Autodesk Inventor part; units mm, degrees
ref_plane "ANBAU_XY" through (0, 0, 0) normal (0, 0, 1) x (1, 0, 0)
ref_plane "ANBAU_YZ" through (0, 0, 0) normal (1, 0, 0) x (0, 1, 0)
ref_plane "ANBAU_ZX" through (0, 0, 0) normal (0, 1, 0) x (0, 0, 1)
sketch "Sketch_1" plane through (0, 0, 0) normal (1, 0, 0) x (0, 1, 0)
  line L0 (0, -19) -> (0, 0)
  line L1 (23, 0) -> (23, -8.65)
  arc A0 (22.6, -9.05) -> (23, -8.65) centre (22.6, -8.65) ccw
  line L2 (22.6, -9.05) -> (16.6, -9.05)
  line L3 (16.6, -9.05) -> (16, -9.65)
  line L4 (16, -9.65) -> (16, -19)
  line L5 (16, -19) -> (37.4, -19)
  line L6 (37.4, -19) -> (39, -17.4)
  line L7 (39, -17.4) -> (39, 0)
  line L8 (39, 0) -> (23, 0)
revolve "Revolution1" add sketch "Sketch_1" angle 360 about axis through (0, 0, -19) along (0, 0, -1)
sketch "Sketch_2" plane through (0, 0, 0) normal (1, 0, 0) x (0, 1, 0)
  line L0 (31, -19) -> (31, 0)
  line L1 (31, 0) -> (37, 0)
  line L2 (37, 0) -> (36.053, -0.947)
  line L3 (36.053, -0.947) -> (36.053, -18.053)
  line L4 (36.053, -18.053) -> (37, -19)
  line L5 (37, -19) -> (31, -19)
  line L6 (31, -19) -> (31, 0)
revolve "Revolution2" cut sketch "Sketch_2" angle 360 about axis through (0, 31, -19) along (0, 0, -1)
thread "Thread1"
pattern_linear "Rectangular Pattern1" count 2 spacing 43.8406 along (-0.7071, -0.7071, 0) count 2 spacing 43.8406 along (0.7071, -0.7071, 0) of "Revolution2"
ref_plane "ANBAU_XY" through (0, 0, 0) normal (0, 0, 1) x (1, 0, 0)
ref_plane "ANBAU_YZ" through (0, 0, 0) normal (1, 0, 0) x (0, 1, 0)
ref_plane "ANBAU_ZX" through (0, 0, 0) normal (0, 1, 0) x (0, 0, 1)
ref_plane "EP_IP_XY" through (0, 0, -9.05) normal (0, 0, -1) x (1, 0, 0)
ref_plane "EP_IP_YZ" through (0, 0, -9.05) normal (1, 0, 0) x (0, -1, 0)
ref_plane "EP_IP_ZX" through (0, 0, -9.05) normal (0, -1, 0) x (0, 0, -1)
properties part number "1559396 EAGF-V2-KF-100---(R)"
The listing builds one solid part. Answer for the finished solid, in the listing's coordinates (mm). A direction names the side the tool comes from. Coordinates: 2 decimals unless noted, no trailing zeros. Loops run counter-clockwise (first coordinate to the right, second up) from the corner with the lowest first, then second, coordinate; pieces in that order, holes last. Notation, with made-up numbers: (73, 33.5) -> (122, 33.5) arc R19 cw to (122, 43.5) -> close; hole circle Ø2 at (86.5, 61.25). An arc over 180 degrees is marked (long way). Write item = value, one per line. Start each with the question number.
1) The mould has two halves that part along Y. Classify faces 1 (the face through (-17, 17, 0)), 2 (the face through (-35.5, 2.3, -9.6)), 3 (the face through (-38.668, -5.077, -8.578)): released by +Y, released by -Y, zero draft, split by the parting line, or undercut.
2) Straight lines are drawn through the part: line 1 (X direction, y = 0, z = -12.75); line 2 (X direction, y = 4, z = -4.75); line 3 (Y direction, x = 5.5, z = -13). For each, find the intervals that lie inside material, in ascending order. Write a range as from..to.
3) Given pin 1 Ø8 at (x, y) = (0, -31) entering from +Z; pin 2 Ø11.5 at (x, y) = (0, 31) entering from -Z; pin 3 Ø1.5 at (y, z) = (-10, -15) entering from -X; pin 4 Ø1.5 at (x, y) = (-2.5, -20) entering from +Z, each flat-ended and moving along its own axis, determine where each tip first touches the part or whether it passes through.
4) A cutting plane is placed at D-D (z = -5.5). Give the vertices of the cut face in (x, y), then the cut area to 3 significant figures.
5) A cutting plane is placed at C-C (z = -11.25). Give the vertices of the cut face in (x, y).
6) A cutting plane is placed at A-A (x = 0). Count the separate pieces of the cut face and the enclosed holes in it, then the cut area to 3 significant figures.
7) A tool of negligible diameter and unlimited length cuts with its end or side. For faces 4 (the face through (12, -12, -9.05)), 5 (the face through (1.52, -26.18, -9.62)), from which of +Z, -Z, +X, -X, +Y, -Y can it reach the whole face along a straight path? Write none if from no direction.
Responses:
q1.face_1 = zero draft
q1.face_2 = undercut
q1.face_3 = split by the parting line
q2.line_1 = -39..-36.05, -25.95..-16, 16..25.95, 36.05..39
q2.line_2 = -38.79..-34.09, -27.91..-22.65, 22.65..27.91, 34.09..38.79
q2.line_3 = -38.61..-15.02, 15.02..38.61
q3.pin_1 = through
q3.pin_2 = -18.75
q3.pin_3 = -37.89
q3.pin_4 = -9.05
q4.outline = circle Ø78 at (0, 0); hole circle Ø10.11 at (-31, 0); hole circle Ø46 at (0, 0); hole circle Ø10.11 at (0, -31); hole circle Ø10.11 at (0, 31); hole circle Ø10.11 at (31, 0)
q4.area = 2,800 mm²
q5.outline = circle Ø78 at (0, 0); hole circle Ø10.11 at (-31, 0); hole circle Ø32 at (0, 0); hole circle Ø10.11 at (0, -31); hole circle Ø10.11 at (0, 31); hole circle Ø10.11 at (31, 0)
q6.separate_pieces = 4
q6.enclosed_holes = 0
q6.area = 357 mm²
q7.face_4 = +Z
q7.face_5 = +Z, -Z
